```python
from build123d import *

# Parameters (mm, degrees)
SKETCH1_W           = 670
SKETCH1_H           = 70
BOSS_EXTRUDE1_DEPTH = 10
SKETCH2_R           = 6
CUT_EXTRUDE1_DEPTH  = 337.97180891
FILLET1_R           = 35


with BuildPart() as part:
    # Sketch1 → Boss-Extrude1 (new body)
    with BuildSketch(Plane.XY):
        Rectangle(SKETCH1_W, SKETCH1_H)
    extrude(amount=BOSS_EXTRUDE1_DEPTH)

    # Sketch2 → Cut-Extrude1 (cut, through all)
    with BuildSketch(Plane.XY.offset(10)):
        with Locations((-300, 0)):
            Circle(SKETCH2_R)
        with Locations((300, 0)):
            Circle(SKETCH2_R)
    extrude(amount=-CUT_EXTRUDE1_DEPTH, mode=Mode.SUBTRACT)

    # Fillet1
    fillet1_edges = [part.edges().sort_by_distance(p)[0] for p in [
        (335, -35, 5),
        (335, 35, 5),
        (-335, -35, 5),
        (-335, 35, 5),
    ]]
    fillet(fillet1_edges, radius=FILLET1_R - 0.0001)  # a hair under: the kernel refuses the full size


solid = part.part
```
Check sheet for the modelled part. Datum: model origin and axes. Units: mm. Give positions to 0.01 mm unless a question says otherwise; leave off trailing zeros. Write each loop counter-clockwise with the first axis right and the second up, starting at its lowest first coordinate (ties: lowest second). Pieces come first, ordered by that corner, then holes. Notation, with made-up numbers: (-14.5, -1.75) - (30.5, -1.75) arc R27 cw to (30.5, 31.25) - close; hole circle Ø1 at (74.5, -40). An arc over 180 degrees is marked (long way). Answer as a JSON object with one key per item and string values. Group by question number.
1) Sectioned sample at B-B (y = 20). Record the cut outline in (x, z).
2) Sectioned sample at A-A (z = 5.5). Give the number of separate pieces and of enclosed holes in the cut face, then the cut area to 3 significant figures.
3) Thickness scan on probe 1 along Y at (x, z) = (-300, 7.75); probe 2 along X at (y, z) = (28, 1); probe 3 along X at (y, z) = (-16, 6.5). Record the ranges inside material, lowest first. Write a range as from..to.
4) Release check for a two-part mould opening along X. For faces 1 (the face through (305.723, 1.802, 5.07)), 2 (the face through (324.475, -25.019, 5.07)), 3 (the face through (-325.019, 24.475, 5.07)), 4 (the face through (-294.277, 1.802, 5.07)) record: pulls with the +X half, pulls with the -X half, needs draft (parallel to the pull), parting line crosses it, or undercut.
5) Depth check by flat-ended pin: P1, Ø1, axis at y = -27, z = 7.5, coming from the -X side; P2, Ø9.5, axis at x = -300, y = 0, coming from the -Z side; P3, Ø2, axis at y = 6, z = 2.5, coming from the +X side. Enter the tip coordinate at first touch or a pass-through.
Geometry results:
{
 "1": {"outline": "(-328.72, 0) - (328.72, 0) - (328.72, 10) - (-328.72, 10) - close"},
 "2": {"separate pieces": "1", "enclosed holes": "2", "area": "45,600 mm^2"},
 "3": {"probe 1": "y = -35..-6, 6..35", "probe 2": "x = -321..321", "probe 3": "x = -331.13..331.13"},
 "4": {"face 1": "undercut", "face 2": "pulls with the +X half", "face 3": "pulls with the -X half", "face 4": "undercut"},
 "5": {"P1": "stops at x = -322.86", "P2": "passes through", "P3": "stops at x = 334.64"}
}
